```python
from build123d import *

# Parameters (mm, degrees)
F0_R     = 9.525
F1_DEPTH = 11.43
F2_R     = 11.43
F3_DEPTH = 177.8
F4_R     = 22.225
F5_DEPTH = 12.7
F6_R     = 5.08
F7_R     = 0.635


with BuildPart() as f1:
    # F0 (on Top) → F1 (new body)
    with BuildSketch(Plane.XY):
        Circle(F0_R)
    extrude(amount=F1_DEPTH)

    # F2 (on face) → F3 (join)
    with BuildSketch(Plane.XY.offset(11.43)):
        Circle(F2_R)
    extrude(amount=F3_DEPTH)

    # F4 (on face) → F5 (join)
    with BuildSketch(Plane.XY.offset(189.23)):
        Circle(F4_R)
    extrude(amount=F5_DEPTH)

    # F6
    f6_edges = [f1.edges().sort_by_distance(p)[0] for p in [
        (-22.225, 0, 201.93),
        (-22.225, 0, 189.23),
    ]]
    fillet(f6_edges, radius=F6_R)

    # F7
    f7_edges = [f1.edges().sort_by_distance(p)[0] for p in [
        (-11.43, 0, 11.43),
        (-9.525, 0, 0),
    ]]
    fillet(f7_edges, radius=F7_R)


solid = f1.part
```
CAD build for the part. Positions are in the model's coordinates, mm. A direction names the side the tool comes from. Round coordinates to 2 decimals unless told otherwise and drop trailing zeros. Loops run counter-clockwise (first coordinate to the right, second up) from the corner with the lowest first, then second, coordinate; pieces in that order, holes last. Notation, with made-up numbers: M 56.5,44.25 L 109.5,44.25 A8 ccw 109.5,58.25 Z; hole C 78.25,57.25 d2. An arc over 180 degrees is marked long. Use a Markdown table: item, result. Add a question column.
(1) Which spindle directions (+Z, -Z, +X, -X, +Y, -Y) get a long thin tool onto all of the face, cutting with end or side? Do faces 1 (the face through (-7.559, -5.796, 5.957)), 2 (the face through (0, 0, 201.93)). Say none if no direction does.
(2) Flat gauge pins, fed straight in: pin 1 (12 mm diameter, centred on y = 14.5, z = 93, fed in from +X); pin 2 (4 mm diameter, centred on x = 17, y = 2, fed in from -Z); pin 3 (4 mm diameter, centred on y = 4.5, z = 159.5, fed in from +X); pin 4 (3 mm diameter, centred on y = 14, z = 34.5, fed in from -X). Where does each tip first touch, or does it go through?
(3) Cut at A-A (x = 0). Give the cut face in (y, z) (3 decimals).
(4) Cut at C-C (z = 37.5). Give the cut face in (x, y).
(5) Drill centre lines: line 1 (Z direction, x = -2.5, y = -17); line 2 (Z direction, x = 7.5, y = -16); line 3 (X direction, y = -0.5, z = 29). Where is each one in solid material? Low to high.
Geometry says:
| question | item | result |
|---|---|---|
| 1 | face 1 | -Z |
| 1 | face 2 | +Z, +X, -X, +Y, -Y |
| 2 | pin 1 | stops at x = 7.64 |
| 2 | pin 2 | stops at z = 189.23 |
| 2 | pin 3 | stops at x = 11.15 |
| 2 | pin 4 | passes through |
| 3 | outline | M -22.225,194.31 A5.08 ccw -17.145,189.23 L -11.43,189.23 L -11.43,12.065 A0.635 ccw -10.795,11.43 L -9.525,11.43 L -9.525,0.635 A0.635 ccw -8.89,0 L 8.89,0 A0.635 ccw 9.525,0.635 L 9.525,11.43 L 10.795,11.43 A0.635 ccw 11.43,12.065 L 11.43,189.23 L 17.145,189.23 A5.08 ccw 22.225,194.31 L 22.225,196.85 A5.08 ccw 17.145,201.93 L -17.145,201.93 A5.08 ccw -22.225,196.85 Z |
| 4 | outline | C 0,0 d22.86 |
| 5 | line 1 | z = 189.23 to 201.93 |
| 5 | line 2 | z = 189.26 to 201.9 |
| 5 | line 3 | x = -11.42 to 11.42 |
